Can you work these out from the model? Positions are in its coordinate system, mm. A direction names the side the tool comes from. Round coordinates to 2 decimals unless told otherwise and drop trailing zeros. Loops run counter-clockwise (first coordinate to the right, second up) from the corner with the lowest first, then second, coordinate; pieces in that order, holes last. Notation, with made-up numbers: M 1,49 L 22,49 A22 cw 22,87 Z; hole C 66,34 d5. An arc over 180 degrees is marked long. Use a Markdown table: item, result. Add a question column.
Autodesk Inventor part; units mm, degrees
ref_plane "YZ Plane" through (0, 0, 0) normal (1, 0, 0) x (0, 1, 0)
ref_plane "XZ Plane" through (0, 0, 0) normal (0, 1, 0) x (-1, 0, 0)
ref_plane "XY Plane" through (0, 0, 0) normal (0, 0, 1) x (1, 0, 0)
sketch "Sketch1" plane through (0, 0, 0) normal (0, 1, 0) x (-1, 0, 0)
  line L0 (-5.7, 11.75) -> (5.7, 11.75) construction
  line L1 (5.7, 11.75) -> (5.7, -11.75) construction
  line L2 (5.7, -11.75) -> (-5.7, -11.75) construction
  line L3 (-5.7, -11.75) -> (-5.7, 11.75) construction
  line L4 (0, 15.7993) -> (0, -16.2311) construction
  line L5 (0, 0) -> (13.9659, 0) construction
  line L6 (-5.7, 16.15) -> (5.7, 16.15) construction
  line L7 (5.7, 16.15) -> (5.7, -16.15) construction
  line L8 (5.7, -16.15) -> (-5.7, -16.15) construction
  line L9 (-5.7, -16.15) -> (-5.7, 16.15) construction
  circle A0 centre (-2.7, 14.15) radius 1.3
  line L10 (0, 0) -> (-13.9659, 0) construction
  circle A1 centre (2.7, 14.15) radius 1.3
  circle A2 centre (-2.7, -14.15) radius 1.3
  circle A3 centre (2.7, -14.15) radius 1.3
  line L11 (-20, 20) -> (20, 20)
  line L12 (20, 20) -> (20, -20)
  line L13 (20, -20) -> (-20, -20)
  line L14 (-20, -20) -> (-20, 20)
  line L15 (0, 0) -> (0, 9.3177) construction
  line L16 (-5.9, 11.95) -> (5.9, 11.95)
  line L17 (5.9, 11.95) -> (5.9, -11.95)
  line L18 (5.9, -11.95) -> (-5.9, -11.95)
  line L19 (-5.9, -11.95) -> (-5.9, 11.95)
  dimension "d1" = 3
  dimension "d2" = 4.4
  dimension "d4" = 23.5
  dimension "d5" = 11.4
  dimension "d6" = 2.6
  dimension "d7" = 40
  dimension "d10" = 0.2
  dimension "d11" = 0.2
  dimension "d14" = 2.4
extrude "Extrusion2" add sketch "Sketch1" along normal blind 1.9
equation "\"d1\" = ServoEdgeToFixation"
equation "\"d2\" = ServoFixationLength"
equation "\"d4\" = ServoCoreLength"
equation "\"d5\" = ServoCoreWidth"
equation "\"d6\" = ServoScrewDiameterRequired"
equation "\"d10\" = ServoTraceSpacing"
equation "\"d11\" = ServoTraceSpacing"
equation "\"d14\" = ServoCoreToFixation"
equation "\"d12\" = ServoArmThickness"
equation "\"ServoTraceSpacing\" = 0.2"
properties part number "ServoTrace"
(1) Suppose I cut it at A-A on z = 14.15. List the corners of the cut face in (x, y) for me.
(2) I'm going to push a flat-ended pin straight in: pin 1 (2 mm diameter, centred on x = 2.7, z = -14.15, fed in from -Y). Where does the tip first touch, or does it pass through?
(3) Suppose I cut it at D-D on y = 1.25. List the corners of the cut face in (x, z) for me, and give its area (3 significant figures).
(4) Suppose I cut it at B-B on x = 2.7. List the corners of the cut face in (y, z) for me.
(5) On a 3-axis mill with a long thin cutter (end or side, diameter ignored), from which of +Z, -Z, +X, -X, +Y, -Y can I reach the whole of each face in a straight line? I mean faces 1 (the face through (0, 1, -20)), 2 (the face through (5.9, 1, 0)). Say none if no direction works.
(6) Thinking about a two-plate mould opening in X: for faces 3 (the face through (-9, 1.9, 0)), 4 (the face through (20, 1, 0)), 5 (the face through (-3.9, 0.94, -13.65)), which applies, released by +X, released by -X, zero draft, split by the parting line, or undercut?
(7) If I drill on probe 1 along X at (y, z) = (1.3, -14); probe 2 along Z at (x, y) = (2.7, 0.8); probe 3 along Z at (x, y) = (3.5, 1.8), over which ranges is the centre line in solid material (lowest first)? Write a range as [from, to].
(8) Suppose I cut it at C-C on z = 2. List the corners of the cut face in (x, y) for me, and give its area (3 significant figures).
Results below:
| question | item | result |
|---|---|---|
| 1 | outline | M -20,0 L -4,0 L -4,1.9 L -20,1.9 Z; M -1.4,0 L 1.4,0 L 1.4,1.9 L -1.4,1.9 Z; M 4,0 L 20,0 L 20,1.9 L 4,1.9 Z |
| 2 | pin 1 | passes through |
| 3 | outline | M -20,-20 L 20,-20 L 20,20 L -20,20 Z; hole M -5.9,-11.95 L 5.9,-11.95 L 5.9,11.95 L -5.9,11.95 Z; hole C -2.7,-14.15 d2.6; hole C -2.7,14.15 d2.6; hole C 2.7,-14.15 d2.6; hole C 2.7,14.15 d2.6 |
| 3 | area | 1,300 mm² |
| 4 | outline | M 0,-20 L 1.9,-20 L 1.9,-15.45 L 0,-15.45 Z; M 0,-12.85 L 1.9,-12.85 L 1.9,-11.95 L 0,-11.95 Z; M 0,11.95 L 1.9,11.95 L 1.9,12.85 L 0,12.85 Z; M 0,15.45 L 1.9,15.45 L 1.9,20 L 0,20 Z |
| 5 | face 1 | -Z, +X, -X, +Y, -Y |
| 5 | face 2 | +Y, -Y |
| 6 | face 3 | zero draft |
| 6 | face 4 | released by +X |
| 6 | face 5 | undercut |
| 7 | probe 1 | x = [-20, -3.99], [-1.41, 1.41], [3.99, 20] |
| 7 | probe 2 | z = [-20, -15.45], [-12.85, -11.95], [11.95, 12.85], [15.45, 20] |
| 7 | probe 3 | z = [-20, -15.17], [-13.13, -11.95], [11.95, 13.13], [15.17, 20] |
| 8 | outline | M -20,0 L -5.9,0 L -5.9,1.9 L -20,1.9 Z; M 5.9,0 L 20,0 L 20,1.9 L 5.9,1.9 Z |
| 8 | area | 53.6 mm² |
